```python
from build123d import *

# Parameters (mm, degrees)
HEX_EXTRUDE_DEPTH      = 58.145
MOTOR_SHAFT_DEPTH      = 9
SKETCH15_R             = 5.666174209
SKETCH15_R_2           = 2.2
MOTOR_SPACER_DEPTH     = 1.6
SKETCH16_R             = 5.666174209
HUB_INNER_SPACER_DEPTH = 7.76
SKETCH14_R             = 1.95
BEARING_DEPTH          = 3.048


with BuildPart() as part:
    # Standoff → Hex extrude (new body)
    with BuildSketch(Plane.XY.offset(1.6)):
        Polygon((3.666174209, 0), (1.833087105, 3.175), (-1.833087105, 3.175), (-3.666174209, 0), (-1.833087105, -3.175), (1.833087105, -3.175), align=None)
    extrude(amount=HEX_EXTRUDE_DEPTH)

    # Sketch12 → Motor shaft (cut)
    with BuildSketch(Plane.XY.offset(1.6)):
        with BuildLine():
            Line((1.394668419, 1.57), (-1.394668419, 1.57))
            ThreePointArc((-1.394668419, 1.57), (0, -2.1), (1.394668419, 1.57))
        make_face()
    extrude(amount=MOTOR_SHAFT_DEPTH, mode=Mode.SUBTRACT)

    # Sketch15 → Motor spacer (add)
    with BuildSketch(Plane.XY):
        Circle(SKETCH15_R)
        Circle(SKETCH15_R_2, mode=Mode.SUBTRACT)
    extrude(amount=MOTOR_SPACER_DEPTH)

    # Sketch16 → Hub inner spacer (add)
    with BuildSketch(Plane.XY.offset(1.6)):
        with Locations(Location((0, 0, 0), (0, 0, 180))):
            Circle(SKETCH16_R)
        Polygon((3.666174209, 0), (1.833087105, 3.175), (-1.833087105, 3.175), (-3.666174209, 0), (-1.833087105, -3.175), (1.833087105, -3.175), align=None, mode=Mode.SUBTRACT)
    extrude(amount=HUB_INNER_SPACER_DEPTH)

    # Sketch14 → Bearing (add)
    with BuildSketch(Plane.XY.offset(59.745)):
        with Locations(Location((0, 0, 0), (0, 0, 270))):
            Circle(SKETCH14_R)
    extrude(amount=BEARING_DEPTH)


solid = part.part
```
Geometry: final body of the model. Coordinates: model frame, mm. A direction names the side the tool comes from. Coordinates: 2 decimals unless noted, no trailing zeros. Write each loop counter-clockwise with the first axis right and the second up, starting at its lowest first coordinate (ties: lowest second). Pieces come first, ordered by that corner, then holes. Notation, with made-up numbers: M -32.75,-3 L -12.75,-3 A21 ccw -12.75,16 Z; hole C 74.25,84.5 d9. An arc over 180 degrees is marked long. Answer as CSV lines item,"result". Start each with the question number.
Q1. Cut plane D-D on y = -4.75. Return the cut outline in (x, z), then the cut area to 3 significant figures.
Q2. Mould query, pull axis Y, two halves, no side actions, for faces 1 (the flat face through (0, 0, 62.793)), 2 (the flat face through (0, 2, 1.6)), 3 (the cylindrical face through (-1.187, 1.547, 61.248)). Classes: released by +Y, released by -Y, zero draft, split by the parting line, or undercut.
Q3. Reachability of faces 4 (the flat face through (2, 1, 59.745)), 5 (the flat face through (2.76, 1.57, 34.2)), 6 (the cylindrical face through (-0.07, -2.1, 6.04)) from +Z, -Z, +X, -X, +Y, -Y: full face, straight path, thin tool, end or side. Return the list, or none.
Q4. Cut plane C-C on z = 6.5. Return the cut outline in (x, y).
Q5. Cut plane A-A on z = 46.5. Return the cut outline in (x, y) (3 decimals).
Q6. Pin query (flat end, axial travel): P1, Ø2, axis at x = 3, z = 34.5, coming from the -Y side; P2, Ø1.5, axis at x = -0.5, y = -3, coming from the -Z side; P3, Ø1.1, axis at x = -1, y = 0, coming from the -Z side; P4, Ø4, axis at x = 4.5, y = -4, coming from the +Z side. Return the tip coordinate at first contact, or that it passes through.
Q7. Line query: line 1 (Y direction, x = 0, z = 0.9); line 2 (Y direction, x = -1.25, z = 48) (3 decimals); line 3 (Z direction, x = 1.5, y = -1.5) (3 decimals). Output: solid intervals per line, ascending. Write a range as from..to.
Q8. Cut plane B-B on y = -1. Return the cut outline in (x, z) (3 decimals).
Findings below:
1,outline,"M -3.09,0 L 3.09,0 L 3.09,9.36 L -3.09,9.36 Z"
1,area,"57.8 mm2"
2,face 1,"zero draft"
2,face 2,"undercut"
2,face 3,"split by the parting line"
3,face 4,"+Z"
3,face 5,"+Z, +X, +Y"
3,face 6,"-Z"
4,outline,"C 0,0 d11.33; hole M -1.39,1.57 A2.1 ccw long 1.39,1.57 Z"
5,outline,"M -3.666,0 L -1.833,-3.175 L 1.833,-3.175 L 3.666,0 L 1.833,3.175 L -1.833,3.175 Z"
6,P1,"stops at y = -2.89"
6,P2,"stops at z = 0"
6,P3,"stops at z = 10.6"
6,P4,"stops at z = 9.36"
7,line 1,"y = -5.67..-2.2, 2.2..5.67"
7,line 2,"y = -3.175..3.175"
7,line 3,"z = 1.6..59.745"
8,outline,"M -5.577,0 L -1.96,0 L -1.96,1.6 L -1.847,1.6 L -1.847,10.6 L 1.847,10.6 L 1.847,1.6 L 1.96,1.6 L 1.96,0 L 5.577,0 L 5.577,9.36 L 3.089,9.36 L 3.089,59.745 L 1.674,59.745 L 1.674,62.793 L -1.674,62.793 L -1.674,59.745 L -3.089,59.745 L -3.089,9.36 L -5.577,9.36 Z"
